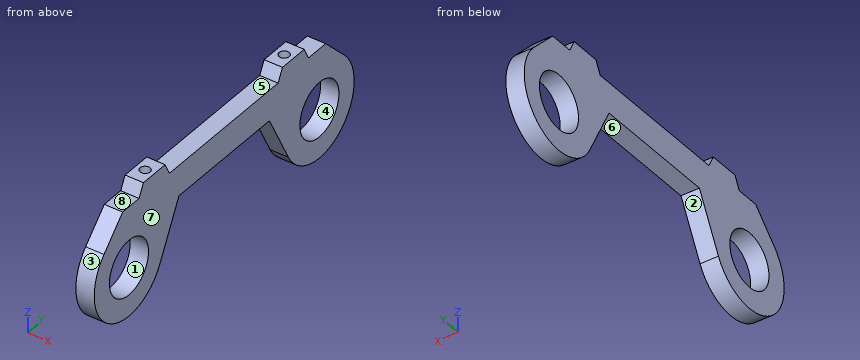
Autodesk Inventor part; units mm, degrees
ref_plane "Work Plane2" through (0, -64.0035, 48.0084) normal (0, 0, 1) x (1, 0, 0)
ref_plane "YZ Plane" through (0, 0, 0) normal (1, 0, 0) x (0, 1, 0)
ref_plane "XZ Plane" through (0, 0, 0) normal (0, 1, 0) x (-1, 0, 0)
sketch "Sketch1" plane through (0, 0, 0) normal (1, 0, 0) x (0, 1, 0)
  arc A0 (59.469, -14.4909) -> (110.9653, 22.2844) centre (87.9998, 0.0002) ccw
  line L0 (110.9653, 22.2844) -> (93.7688, 40.0067)
  line L1 (0.3424, 140.3326) -> (0.3424, -179.6674) construction
  arc A1 (-110.2805, 22.2844) -> (-58.7842, -14.4909) centre (-87.315, 0.0002) ccw
  line L2 (-110.2805, 22.2844) -> (-93.0839, 40.0067)
  line L3 (-88, 40.0067) -> (-88.0045, 40)
  line L4 (57.9955, 40) -> (58, 40.0067)
  line L5 (49.9965, 40.0151) -> (-50.0337, 40.0151)
  line L6 (59.469, -14.4909) -> (41.9609, 19.9801)
  line L7 (-58.7842, -14.4909) -> (-41.2761, 19.9801)
  line L8 (41.9609, 19.9801) -> (-41.2761, 19.9801)
  line L9 (78, 40.0067) -> (73.9965, 48.0084)
  line L10 (73.9965, 48.0084) -> (53.9965, 48.0084)
  line L11 (53.9965, 48.0084) -> (49.9965, 40.0151)
  line L12 (-78, 40.0067) -> (-74.0035, 48.0084)
  line L13 (-74.0035, 48.0084) -> (-54.0035, 48.0084)
  line L14 (-54.0035, 48.0084) -> (-50.0337, 40.0151)
  line L15 (93.7688, 40.0067) -> (78, 40.0067)
  line L16 (-78, 40.0067) -> (-93.0839, 40.0067)
  point P0 (0, 0)
  point P1 (83, 40)
  point P2 (63.9965, 48.0084)
  point P3 (-64.0035, 48.0084)
extrude "Extrusion2" add sketch "Sketch1" along normal blind 12
hole "Hole4" at (0, -87.315, 0.0002) at (0, 87.9998, 0.0002) direction (1, 0, 0) diameter 36 end through all
ref_plane "Work Plane2" through (0, -64.0035, 48.0084) normal (0, 0, 1) x (1, 0, 0)
sketch "Sketch3" plane through (0, -74.0035, 48.0084) normal (0, 0, 1) x (1, 0, 0)
  point P0 (0, 74.0035)
  point P1 (6, 10)
  point P2 (6, 138)
hole "Hole5" at (6, -64.0035, 48.0084) at (6, 63.9965, 48.0084) direction (0, 0, -1) diameter 6.647 depth 20 tip angle 118
properties part number "PlateConnector"
Geometry check sheet. Reference: the model listing, model coordinates, mm. Face numbers are marked on the shaded views. A direction names the side the tool comes from. Give positions to 0.01 mm unless a question says otherwise; leave off trailing zeros. Order: outer loops, then holes, each group sorted by start corner. A loop starts at its lowest first (then second) coordinate and runs counter-clockwise, first axis right, second up.
1. Section check D-D, the plane y = 57. Enter the section's corners in (x, z), and give its area (3 significant figures).
2. Access from +Z, -Z, +X, -X, +Y, -Y to the whole of each face (thin tool, end or side, straight path). Record for the marked faces 4, 5, 6, 7 and 8.
3. Release check for a two-part mould opening along Z. For the marked faces 1, 2 and 3 record: pulls with the +Z half, pulls with the -Z half, needs draft (parallel to the pull), parting line crosses it, or undercut.
4. Section check B-B, the plane y = 101.5. Enter the section's corners in (x, z).
5. Section check C-C, the plane z = -10.5. Enter the section's corners in (x, y), and give its area (3 significant figures).
6. Thickness scan on L1, parallel to Y at x = 6, z = 41; L2, parallel to Y at x = 9, z = 6.5; L3, parallel to Y at x = 7.5, z = 37.5. Record the ranges inside material, lowest first.
7. Section check A-A, the plane z = 11.5. Enter the section's corners in (x, y).
8. Gauge pin test, flat ends, axial feed: pin 1 Ø1.5 at (x, y) = (10.5, -6) entering from -Z; pin 2 Ø4 at (x, z) = (8, 15.5) entering from -Y; pin 3 Ø2 at (x, y) = (2, 50) entering from +Z. Record the tip position at first contact, or that the pin passes through.
Values follow:
1. outline: (0, -9.63) - (12, -9.63) - (12, 48.01) - (0, 48.01) - close
1. area: 692 mm2
2. face 4: +X, -X
2. face 5: +Z, +X, -X
2. face 6: -Z, +X, -X
2. face 7: +Z, -Z, +X, +Y, -Y
2. face 8: +Z, +X, -X, -Y
3. face 1: undercut
3. face 2: pulls with the -Z half
3. face 3: parting line crosses it
4. outline: (0, -29.01) - (12, -29.01) - (12, -11.91) - (0, -11.91) - close; (0, 11.91) - (12, 11.91) - (12, 32.04) - (0, 32.04) - close
5. outline: (0, -117.54) - (12, -117.54) - (12, -101.94) - (0, -101.94) - close; (0, -72.69) - (12, -72.69) - (12, -56.76) - (0, -56.76) - close; (0, 57.44) - (12, 57.44) - (12, 73.38) - (0, 73.38) - close; (0, 102.62) - (12, 102.62) - (12, 118.23) - (0, 118.23) - close
5. area: 757 mm2
6. L1: y = -77.5 to -67.33, -60.68 to -50.52, 50.49 to 60.67, 67.32 to 77.5
6. L2: y = -118.65 to -104.1, -70.53 to -48.12, 48.81 to 71.21, 104.79 to 119.33
6. L3: y = -95.52 to -66.97, -61.04 to 61.03, 66.96 to 96.2
7. outline: (0, -117.18) - (12, -117.18) - (12, -101.16) - (0, -101.16) - close; (0, -73.47) - (12, -73.47) - (12, -45.58) - (0, -45.58) - close; (0, 46.27) - (12, 46.27) - (12, 74.15) - (0, 74.15) - close; (0, 101.85) - (12, 101.85) - (12, 117.86) - (0, 117.86) - close
8. pin 1: stops at z = 19.98
8. pin 2: stops at y = -116.33
8. pin 3: stops at z = 42.02
